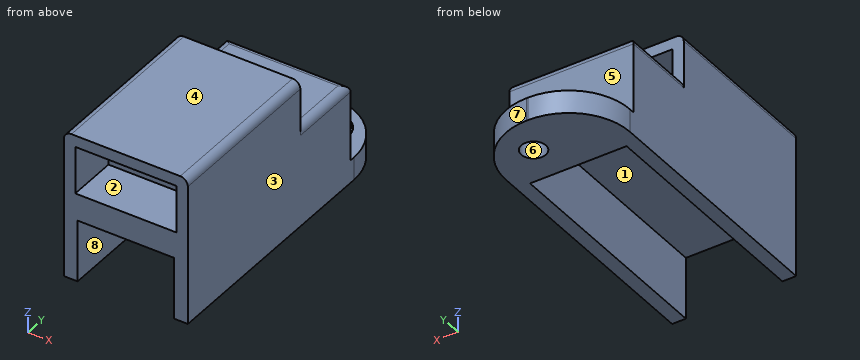
from build123d import *

# Parameters (mm, degrees)
CROQUIS2_W               = 16.2
CROQUIS2_H               = 9.2
CROQUIS2_W_2             = 13.2
CROQUIS2_H_2             = 6.2
SALIENTE_EXTRUIR1_DEPTH  = 6.5
CROQUIS3_W               = 16.2
CROQUIS3_H               = 12
SALIENTE_EXTRUIR2_DEPTH  = 2
SALIENTE_EXTRUIR3_DEPTH  = 8.1
CROQUIS5_W               = 16.2
CROQUIS5_H               = 3
SALIENTE_EXTRUIR4_DEPTH  = 13
CROQUIS6_R               = 1.6
CORTAR_EXTRUIR1_DEPTH    = 3
CROQUIS7_W               = 16.2
CROQUIS7_H               = 2
SALIENTE_EXTRUIR5_DEPTH  = 3
CROQUIS8_R               = 2.9
CORTAR_EXTRUIR2_DEPTH    = 0.5
REDONDEO1_R              = 1
REDONDEO6_R              = 8
CROQUIS9_W               = 13.2
CROQUIS9_H               = 6.2
SALIENTE_EXTRUIR6_DEPTH  = 3.5
CROQUIS10_W              = 13.2
CROQUIS10_H              = 1.5
SALIENTE_EXTRUIR7_DEPTH  = 3.5
CROQUIS11_W              = 13.2
CROQUIS11_H              = 6.2
SALIENTE_EXTRUIR8_DEPTH  = 12
CROQUIS12_W              = 13.2
CROQUIS12_H              = 1.5
SALIENTE_EXTRUIR9_DEPTH  = 12
CROQUIS13_W              = 16.2
CROQUIS13_H              = 7.85
SALIENTE_EXTRUIR10_DEPTH = 10.1
CROQUIS14_W              = 12.6
CROQUIS14_H              = 6.5
CORTAR_EXTRUIR3_DEPTH    = 8.1
REDONDEO7_R              = 1


with BuildPart() as part:
    # Croquis2 → Saliente-Extruir1 (new body)
    with BuildSketch(Plane(origin=(0, 0, 0), x_dir=(1, 0, 0), z_dir=(0, 1, 0))):
        with Locations((6.6, -3.1)):
            Rectangle(CROQUIS2_W, CROQUIS2_H)
        with Locations((6.6, -3.1)):
            Rectangle(CROQUIS2_W_2, CROQUIS2_H_2, mode=Mode.SUBTRACT)
    extrude(amount=SALIENTE_EXTRUIR1_DEPTH)

    # Croquis3 → Saliente-Extruir2 (add)
    with BuildSketch(Plane(origin=(0, 0, -1.5), x_dir=(-1, 0, 0), z_dir=(0, 0, -1))):
        with Locations((-6.6, 6)):
            Rectangle(CROQUIS3_W, CROQUIS3_H)
    extrude(amount=SALIENTE_EXTRUIR2_DEPTH)

    # Croquis4 → Saliente-Extruir3 (add)
    with BuildSketch(Plane(origin=(0, 0, -3.5), x_dir=(-1, 0, 0), z_dir=(0, 0, -1))):
        Polygon((1.5, 0), (1.5, 12), (-14.7, 12), (-14.7, 0), (-12.9, 0), (-12.9, 11), (-0.3, 11), (-0.3, 0), align=None)
    extrude(amount=SALIENTE_EXTRUIR3_DEPTH)

    # Croquis5 → Saliente-Extruir4 (add)
    with BuildSketch(Plane(origin=(0, 12, 0), x_dir=(1, 0, 0), z_dir=(0, 1, 0))):
        with Locations((6.6, 10.1)):
            Rectangle(CROQUIS5_W, CROQUIS5_H)
    extrude(amount=SALIENTE_EXTRUIR4_DEPTH)

    # Croquis6 → Cortar-Extruir1 (cut)
    with BuildSketch(Plane.XY.offset(-8.6)):
        with Locations((9.1, 20)):
            Circle(CROQUIS6_R)
    extrude(amount=-CORTAR_EXTRUIR1_DEPTH, mode=Mode.SUBTRACT)

    # Croquis7 → Saliente-Extruir5 (add)
    with BuildSketch(Plane.XY.offset(-1.5)):
        with Locations((6.6, 7.5)):
            Rectangle(CROQUIS7_W, CROQUIS7_H)
    extrude(amount=SALIENTE_EXTRUIR5_DEPTH)

    # Croquis8 → Cortar-Extruir2 (cut)
    with BuildSketch(Plane.XY.offset(-8.6)):
        with Locations((9.1, 20)):
            Circle(CROQUIS8_R)
    extrude(amount=-CORTAR_EXTRUIR2_DEPTH, mode=Mode.SUBTRACT)

    # Redondeo1
    redondeo1_edges = [part.edges().sort_by_distance(p)[0] for p in [
        (14.7, 3.25, 7.7),
        (-1.5, 3.25, 7.7),
    ]]
    fillet(redondeo1_edges, radius=REDONDEO1_R)

    # Redondeo6
    redondeo6_edges = [part.edges().sort_by_distance(p)[0] for p in [
        (14.7, 25, -10.1),
        (-1.5, 25, -10.1),
    ]]
    fillet(redondeo6_edges, radius=REDONDEO6_R)

    # Croquis9 → Saliente-Extruir6 (add)
    with BuildSketch(Plane.XZ):
        with BuildLine():
            Line((13.7, 7.7), (-0.5, 7.7))
            ThreePointArc((-0.5, 7.7), (-1.207106781, 7.407106781), (-1.5, 6.7))
            Line((-1.5, 6.7), (-1.5, -11.6))
            Line((-1.5, -11.6), (0.3, -11.6))
            Line((0.3, -11.6), (0.3, -3.5))
            Line((0.3, -3.5), (12.9, -3.5))
            Line((12.9, -3.5), (12.9, -11.6))
            Line((12.9, -11.6), (14.7, -11.6))
            Line((14.7, -11.6), (14.7, 6.7))
            ThreePointArc((14.7, 6.7), (14.407106781, 7.407106781), (13.7, 7.7))
        make_face()
        with Locations((6.6, 3.1)):
            Rectangle(CROQUIS9_W, CROQUIS9_H, mode=Mode.SUBTRACT)
    extrude(amount=SALIENTE_EXTRUIR6_DEPTH)

    # Croquis10 → Saliente-Extruir7 (add)
    with BuildSketch(Plane.XZ.offset(-6.5)):
        with Locations((6.6, 0.75)):
            Rectangle(CROQUIS10_W, CROQUIS10_H)
    extrude(amount=SALIENTE_EXTRUIR7_DEPTH)

    # Croquis11 → Saliente-Extruir8 (add)
    with BuildSketch(Plane.XZ.offset(3.5)):
        with BuildLine():
            Line((13.7, 7.7), (-0.5, 7.7))
            ThreePointArc((-0.5, 7.7), (-1.207106781, 7.407106781), (-1.5, 6.7))
            Line((-1.5, 6.7), (-1.5, -11.6))
            Line((-1.5, -11.6), (0.3, -11.6))
            Line((0.3, -11.6), (0.3, -3.5))
            Line((0.3, -3.5), (12.9, -3.5))
            Line((12.9, -3.5), (12.9, -11.6))
            Line((12.9, -11.6), (14.7, -11.6))
            Line((14.7, -11.6), (14.7, 6.7))
            ThreePointArc((14.7, 6.7), (14.407106781, 7.407106781), (13.7, 7.7))
        make_face()
        with Locations((6.6, 3.1)):
            Rectangle(CROQUIS11_W, CROQUIS11_H, mode=Mode.SUBTRACT)
    extrude(amount=SALIENTE_EXTRUIR8_DEPTH)

    # Croquis12 → Saliente-Extruir9 (add)
    with BuildSketch(Plane.XZ.offset(-3)):
        with Locations((6.6, 0.75)):
            Rectangle(CROQUIS12_W, CROQUIS12_H)
    extrude(amount=SALIENTE_EXTRUIR9_DEPTH)

    # Croquis13 → Saliente-Extruir10 (add)
    with BuildSketch(Plane.XY.offset(-8.6)):
        with Locations((6.6, 12.425)):
            Rectangle(CROQUIS13_W, CROQUIS13_H)
    extrude(amount=SALIENTE_EXTRUIR10_DEPTH)

    # Croquis14 → Cortar-Extruir3 (cut)
    with BuildSketch(Plane(origin=(0, 0, -11.6), x_dir=(-1, 0, 0), z_dir=(0, 0, -1))):
        with Locations((-6.6, 11.75)):
            Rectangle(CROQUIS14_W, CROQUIS14_H)
    extrude(amount=-CORTAR_EXTRUIR3_DEPTH, mode=Mode.SUBTRACT)

    # Redondeo7
    redondeo7_edges = [part.edges().sort_by_distance(p)[0] for p in [
        (6.6, 16.35, 1.5),
        (14.7, 11.425, 1.5),
        (-1.5, 11.425, 1.5),
    ]]
    fillet(redondeo7_edges, radius=REDONDEO7_R)


solid = part.part
The listing builds one solid part. Answer for the finished solid, in the listing's coordinates (mm). Face numbers are marked on the shaded views. A direction names the side the tool comes from. Round coordinates to 2 decimals unless told otherwise and drop trailing zeros. Write each loop counter-clockwise with the first axis right and the second up, starting at its lowest first coordinate (ties: lowest second). Pieces come first, ordered by that corner, then holes. Notation, with made-up numbers: M 35,11 L 43,11 A21 cw 43,49 Z; hole C 6,-33.5 d10. An arc over 180 degrees is marked long. Write each question's results on one line, items separated by ' | '. Start each with the question number.
Item 1: Find section C-C on z = -9.5. Write down the section's boundary in (x, y), and give its area (3 significant figures).
Item 2: Find section D-D on x = 3. Write down the section's boundary in (y, z).
Item 3: Find section B-B on y = -11. Write down the section's boundary in (x, z), and give its area (3 significant figures).
Item 4: Straight lines are drawn through the part: probe 1 along X at (y, z) = (-8.5, -6.25); probe 2 along Z at (x, y) = (10.5, -3.5); probe 3 along Z at (x, y) = (2.25, -10.5). For each, find the intervals that lie inside material, in ascending order.
Item 5: The mould has two halves that part along Y. Classify the marked faces 6, 7 and 8: +Y half, -Y half, draft (parallel to the pull), parting line (faces both ways), or undercut.
Item 6: Given pin 1 Ø4 at (x, y) = (4.5, 12) entering from +Z; pin 2 Ø2.5 at (x, y) = (9.1, 20) entering from +Z; pin 3 Ø3.5 at (x, z) = (7, 5.5) entering from +Y; pin 4 Ø8 at (x, z) = (11, -1.5) entering from +Y, each flat-ended and moving along its own axis, determine where each tip first touches the part or whether it passes through.
Item 7: Which of the six approach directions +Z, -Z, +X, -X, +Y, -Y give full straight-line access (tool end or side, diameter ignored) to the marked faces 1, 2, 3, 4 and 5?
Item 8: Find section A-A on z = 4.5. Write down the section's boundary in (x, y).
Answer block:
1) outline: M -1.5,-15.5 L 0.3,-15.5 L 0.3,15 L 12.9,15 L 12.9,-15.5 L 14.7,-15.5 L 14.7,17 A8 ccw 6.7,25 L 6.5,25 A8 ccw -1.5,17 Z; hole C 9.1,20 d3.2 | area: 236 mm²
2) outline: M -15.5,-3.5 L 15,-3.5 L 15,-11.6 L 24.19,-11.6 L 24.19,-8.6 L 16.35,-8.6 L 16.35,0.5 A1 ccw 15.35,1.5 L -9,1.5 L -9,0 L -15.5,0 Z; M -15.5,6.2 L 6.5,6.2 L 6.5,7.7 L -15.5,7.7 Z
3) outline: M -1.5,-11.6 L 0.3,-11.6 L 0.3,-3.5 L 12.9,-3.5 L 12.9,-11.6 L 14.7,-11.6 L 14.7,6.7 A1 ccw 13.7,7.7 L -0.5,7.7 A1 ccw -1.5,6.7 Z; hole M 0,0 L 13.2,0 L 13.2,6.2 L 0,6.2 Z | area: 128 mm²
4) probe 1: x = -1.5 to 0.3, 12.9 to 14.7 | probe 2: z = -3.5 to 1.5, 6.2 to 7.7 | probe 3: z = -3.5 to 0, 6.2 to 7.7
5) face 6: undercut | face 7: +Y half | face 8: draft
6) pin 1: stops at z = 1.5 | pin 2: passes through | pin 3: stops at y = 6.5 | pin 4: stops at y = 16.35
7) face 1: -Z, -Y | face 2: -Y | face 3: +Z, -Z, +X, +Y, -Y | face 4: +Z, +X, -X, +Y, -Y | face 5: +Z, +X, -X, +Y
8) outline: M -1.5,-15.5 L 0,-15.5 L 0,6.5 L -1.5,6.5 Z; M 13.2,-15.5 L 14.7,-15.5 L 14.7,6.5 L 13.2,6.5 Z
